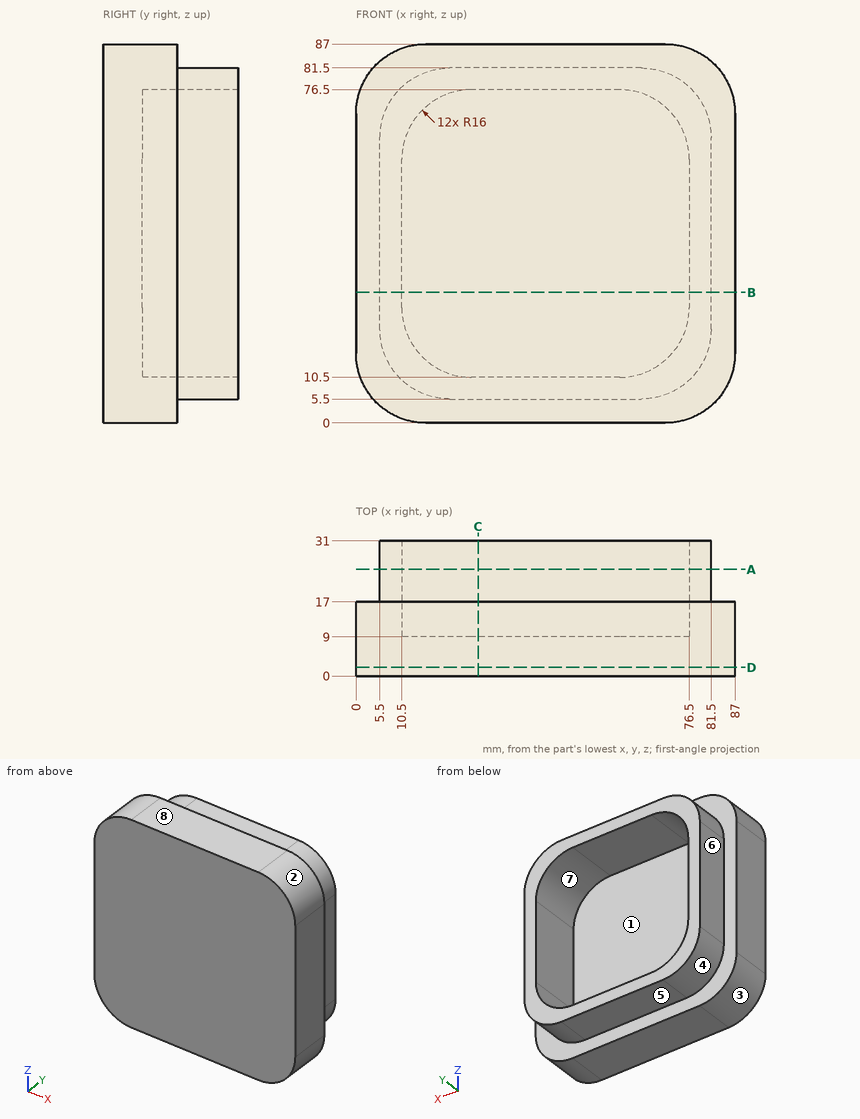
Can you work these out from the drawing? Everything is in mm from the part's minimum corner. A direction names the side the tool comes from. Round coordinates to 2 decimals unless told otherwise and drop trailing zeros. Write each loop counter-clockwise with the first axis right and the second up, starting at its lowest first coordinate (ties: lowest second). Pieces come first, ordered by that corner, then holes. Notation, with made-up numbers: M -35.75,-22 L 21.25,-22 A14 cw 21.25,4 Z; hole C -35.5,-5 d4. An arc over 180 degrees is marked long. Use a Markdown table: item, result.
Item 1: I want a section at D-D (y = 2). List the corners of the cut face in (x, z) for me, and give its area (3 significant figures).
Found:
| item | result |
|---|---|
| outline | M 0,16 A16 ccw 16,0 L 71,0 A16 ccw 87,16 L 87,71 A16 ccw 71,87 L 16,87 A16 ccw 0,71 Z |
| area | 7,350 mm2 |
Item 2: Which directions (+Z, -Z, +X, -X, +Y, -Y) give clear straight access to the entire face, cutting with the end or side of a thin tool? Please do the marked faces 4, 5, 6, 7 and 8.
Found:
| item | result |
|---|---|
| face 4 | -Z, -X, +Y |
| face 5 | -Z, +X, -X, +Y |
| face 6 | +Z, -Z, -X, +Y |
| face 7 | +Y |
| face 8 | +Z, +X, -X, +Y, -Y |
Item 3: I want a section at A-A (y = 24.5). List the corners of the cut face in (x, z) for me.
Found:
| item | result |
|---|---|
| outline | M 5.5,21.5 A16 ccw 21.5,5.5 L 65.5,5.5 A16 ccw 81.5,21.5 L 81.5,65.5 A16 ccw 65.5,81.5 L 21.5,81.5 A16 ccw 5.5,65.5 Z; hole M 10.5,26.5 A16 ccw 26.5,10.5 L 60.5,10.5 A16 ccw 76.5,26.5 L 76.5,60.5 A16 ccw 60.5,76.5 L 26.5,76.5 A16 ccw 10.5,60.5 Z |
Item 4: I want a section at C-C (x = 28). List the corners of the cut face in (y, z) for me, and give its area (3 significant figures).
Found:
| item | result |
|---|---|
| outline | M 0,0 L 17,0 L 17,5.5 L 31,5.5 L 31,10.5 L 9,10.5 L 9,76.5 L 31,76.5 L 31,81.5 L 17,81.5 L 17,87 L 0,87 Z |
| area | 1,090 mm2 |
Item 5: We'd pull the mould along Z, two halves only. Please class the marked faces 1, 2 and 3: released by +Z, released by -Z, zero draft, split by the parting line, or undercut.
Found:
| item | result |
|---|---|
| face 1 | undercut |
| face 2 | released by +Z |
| face 3 | released by -Z |
Item 6: If I drill on line 1 along Z through (x, y) = (59, 18); line 2 along X through (y, z) = (12, 48), over which ranges is the centre line in solid material (lowest first)? Write a range as [from, to].
Found:
| item | result |
|---|---|
| line 1 | z = [5.5, 10.5], [76.5, 81.5] |
| line 2 | x = [0, 10.5], [76.5, 87] |
Item 7: For pin 1 Ø5 at (y, z) = (27.5, 43) entering from +X; pin 2 Ø5 at (x, y) = (36, 22.5) entering from -Z; pin 3 Ø1 at (x, z) = (18, 37) entering from +Y, each with a flat end and sliding along its axis, tell me the tip position at first contact or that it passes through.
Found:
| item | result |
|---|---|
| pin 1 | stops at x = 81.5 |
| pin 2 | stops at z = 5.5 |
| pin 3 | stops at y = 9 |
Item 8: I want a section at B-B (z = 30). List the corners of the cut face in (x, y) for me, and give its area (3 significant figures).
Found:
| item | result |
|---|---|
| outline | M 0,0 L 87,0 L 87,17 L 81.5,17 L 81.5,31 L 76.5,31 L 76.5,9 L 10.5,9 L 10.5,31 L 5.5,31 L 5.5,17 L 0,17 Z |
| area | 1,090 mm2 |
